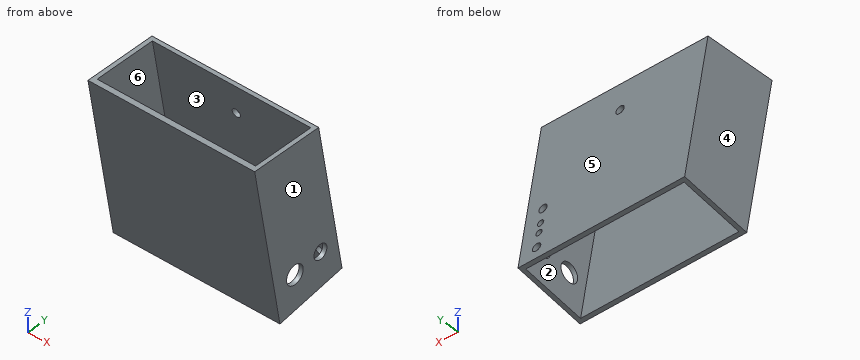
```python
from build123d import *

# Parameters (mm, degrees)
CYLINDER007_R          = 11
CYLINDER007_DEPTH      = 2
CYLINDER012_R          = 2.5
CYLINDER012_DEPTH      = 2
CYLINDER013_R          = 2
CYLINDER013_DEPTH      = 2
CYLINDER014_R          = 3.5
CYLINDER014_DEPTH      = 2
CYLINDER015_R          = 4.5
CYLINDER015_DEPTH      = 2
BOX019_W               = 80
BOX019_H               = 38
BOX019_DEPTH           = 8
BOX019_PLACEMENT_ANGLE = 10
CYLINDER024_R          = 2
CYLINDER024_DEPTH      = 3
CYLINDER025_R          = 2
CYLINDER025_DEPTH      = 2
CYLINDER026_R          = 1.5
CYLINDER026_DEPTH      = 2
CYLINDER027_R          = 1.5
CYLINDER027_DEPTH      = 2
BOX004_W               = 76
BOX004_H               = 30
BOX004_DEPTH           = 78
BOX003_W               = 80
BOX003_H               = 34
BOX003_DEPTH           = 80
CUT012_PLACEMENT_ANGLE = 10


with BuildPart() as basehole:
    # Cylinder007 → Cylinder007 (new body)
    with BuildSketch(Plane(origin=(15, -19, 20), x_dir=(1, 0, 0), z_dir=(0, 0, 1))):
        Circle(CYLINDER007_R)
    extrude(amount=CYLINDER007_DEPTH)


with BuildPart() as volumehole:
    # Cylinder012 → Cylinder012 (new body)
    with BuildSketch(Plane(origin=(62, -20, 20), x_dir=(1, 0, 0), z_dir=(0, 0, 1))):
        Circle(CYLINDER012_R)
    extrude(amount=CYLINDER012_DEPTH)


with BuildPart() as extspeakerhole:
    # Cylinder013 → Cylinder013 (new body)
    with BuildSketch(Plane(origin=(70, 1, -45), x_dir=(1, 0, 0), z_dir=(0, -1, 0))):
        Circle(CYLINDER013_R)
    extrude(amount=CYLINDER013_DEPTH)


with BuildPart() as obj1:
    # Cylinder014 → Cylinder014 (new body)
    with BuildSketch(Plane(origin=(76, -8, -35), x_dir=(0, 0, -1), z_dir=(1, 0, 0))):
        Circle(CYLINDER014_R)
    extrude(amount=CYLINDER014_DEPTH)


with BuildPart() as obj2:
    # Cylinder015 → Cylinder015 (new body)
    with BuildSketch(Plane(origin=(76, -22, -35), x_dir=(0, 0, -1), z_dir=(1, 0, 0))):
        Circle(CYLINDER015_R)
    extrude(amount=CYLINDER015_DEPTH)


with BuildPart() as frontlevel:
    # Box019 → Box019 (new body)
    with BuildSketch(Plane.XY):
        with Locations((40, 19)):
            Rectangle(BOX019_W, BOX019_H)
    extrude(amount=BOX019_DEPTH)


with BuildPart() as frontlevel_1:
    # Box019 placement: moved
    add(frontlevel.part.moved(Location((-2, -36, 28))).rotate(Axis((-2, -36, 28), (-1, 0, 0)), BOX019_PLACEMENT_ANGLE))


with BuildPart() as wirehole002:
    # Cylinder024 → Cylinder024 (new body)
    with BuildSketch(Plane(origin=(38, 1, 7), x_dir=(1, 0, 0), z_dir=(0, -1, 0))):
        Circle(CYLINDER024_R)
    extrude(amount=CYLINDER024_DEPTH)


with BuildPart() as extspeakerhole001:
    # Cylinder025 → Cylinder025 (new body)
    with BuildSketch(Plane(origin=(70, 1, -25), x_dir=(1, 0, 0), z_dir=(0, -1, 0))):
        Circle(CYLINDER025_R)
    extrude(amount=CYLINDER025_DEPTH)


with BuildPart() as extspeakerhole002:
    # Cylinder026 → Cylinder026 (new body)
    with BuildSketch(Plane(origin=(70, 1, -32.5), x_dir=(1, 0, 0), z_dir=(0, -1, 0))):
        Circle(CYLINDER026_R)
    extrude(amount=CYLINDER026_DEPTH)


with BuildPart() as extspeakerhole003:
    # Cylinder027 → Cylinder027 (new body)
    with BuildSketch(Plane(origin=(70, 1, -37.5), x_dir=(1, 0, 0), z_dir=(0, -1, 0))):
        Circle(CYLINDER027_R)
    extrude(amount=CYLINDER027_DEPTH)


with BuildPart() as obj3:
    # Box004 → Box004 (new body)
    with BuildSketch(Plane(origin=(0, -31, -51), x_dir=(1, 0, 0), z_dir=(0, 0, 1))):
        with Locations((38, 15)):
            Rectangle(BOX004_W, BOX004_H)
    extrude(amount=BOX004_DEPTH)

    # Fusion008: union BaseHole, VolumeHole, ExtSpeakerHole, obj1, obj2, FrontLevel, WireHole002, ExtSpeakerHole001, ExtSpeakerHole002, ExtSpeakerHole003
    add(basehole.part)
    add(volumehole.part)
    add(extspeakerhole.part)
    add(obj1.part)
    add(obj2.part)
    add(frontlevel_1.part)
    add(wirehole002.part)
    add(extspeakerhole001.part)
    add(extspeakerhole002.part)
    add(extspeakerhole003.part)


with BuildPart() as base:
    # Box003 → Box003 (new body)
    with BuildSketch(Plane(origin=(-2, -33, -51), x_dir=(1, 0, 0), z_dir=(0, 0, 1))):
        with Locations((40, 17)):
            Rectangle(BOX003_W, BOX003_H)
    extrude(amount=BOX003_DEPTH)

    # Cut012: cut obj3
    add(obj3.part, mode=Mode.SUBTRACT)


with BuildPart() as base_1:
    # Cut012 placement: moved
    add(base.part.rotate(Axis((0, 0, 0), (1, 0, 0)), CUT012_PLACEMENT_ANGLE))


solid = base_1.part
```
Can you work these out from the model? Positions are in its coordinate system, mm. Face numbers are marked on the shaded views. A direction names the side the tool comes from. Coordinates: 2 decimals unless noted, no trailing zeros. Loops run counter-clockwise (first coordinate to the right, second up) from the corner with the lowest first, then second, coordinate; pieces in that order, holes last.
1) Thinking about a two-plate mould opening in Y: for the marked faces 4, 5 and 6, which applies, pulls with the +Y half, pulls with the -Y half, needs draft (parallel to the pull), parting line crosses it, or undercut?
2) Imagine slicing it at A-A on x = 30. List the corners of the cut face in (y, z) for me.
3) Which directions (+Z, -Z, +X, -X, +Y, -Y) give clear straight access to the entire face, cutting with the end or side of a thin tool? Please do the marked faces 1, 2 and 3.
4) For pin 1 (6.5 mm diameter, centred on y = -1.8, z = -35.86, fed in from +X); pin 2 (8 mm diameter, centred on x = 50.5, z = -32, fed in from -Y); pin 3 (8 mm diameter, centred on x = 30.5, z = -14.5, fed in from +Y), each with a flat end and sliding along its axis, tell me the tip position at first contact or that it passes through.
5) I need wall thicknesses on probe 1 along X at (y, z) = (-1, -50.5); probe 2 along Y at (x, z) = (66, 8.5); probe 3 along Y at (x, z) = (56, -24). Which ranges of each line are inside material? Lowest first, please.
6) Imagine slicing it at B-B on y = -17. List the corners of the cut face in (x, z) for me, plus the area to 3 significant figures.
7) Imagine slicing it at C-C on y = -25. List the corners of the cut face in (x, z) for me, plus the area to 3 significant figures.
8) Imagine slicing it at D-D on z = -48.5. List the corners of the cut face in (x, y) for me.
Completed:
1. face 4: needs draft
1. face 5: pulls with the +Y half
1. face 6: undercut
2. outline: (-37.27, 21.32) - (-23.64, -55.96) - (-21.67, -55.61) - (-35.22, 21.21) - (-34.56, 21.32) - close; (-4.78, 21.32) - (7.87, -50.4) - (9.84, -50.05) - (-2.74, 21.32) - close
3. face 1: +Z, -Z, +X, +Y, -Y
3. face 2: none
3. face 3: -Z
4. pin 1: stops at x = 0
4. pin 2: stops at y = -28.57
4. pin 3: stops at y = 4.28
5. probe 1: x = -2 to 0, 76 to 78
5. probe 2: y = -35.01 to -32.98, -2.51 to -0.48
5. probe 3: y = -29.28 to -27.25, 3.22 to 5.25
6. outline: (-2, -54.78) - (0, -54.78) - (0, 21.32) - (-2, 21.32) - close; (76, -54.78) - (78, -54.78) - (78, -42.56) - (76, -42.56) - close; (76, -34.02) - (78, -34.02) - (78, 21.32) - (76, 21.32) - close
6. area: 287 mm2
7. outline: (-2, -48.26) - (78, -48.26) - (78, 21.32) - (76, 21.32) - (76, -36.74) - (0, -36.74) - (0, 21.32) - (-2, 21.32) - close
7. area: 1,150 mm2
8. outline: (-2, -24.96) - (78, -24.96) - (78, 9.57) - (-2, 9.57) - close; hole (0, -22.93) - (76, -22.93) - (76, 7.54) - (0, 7.54) - close
